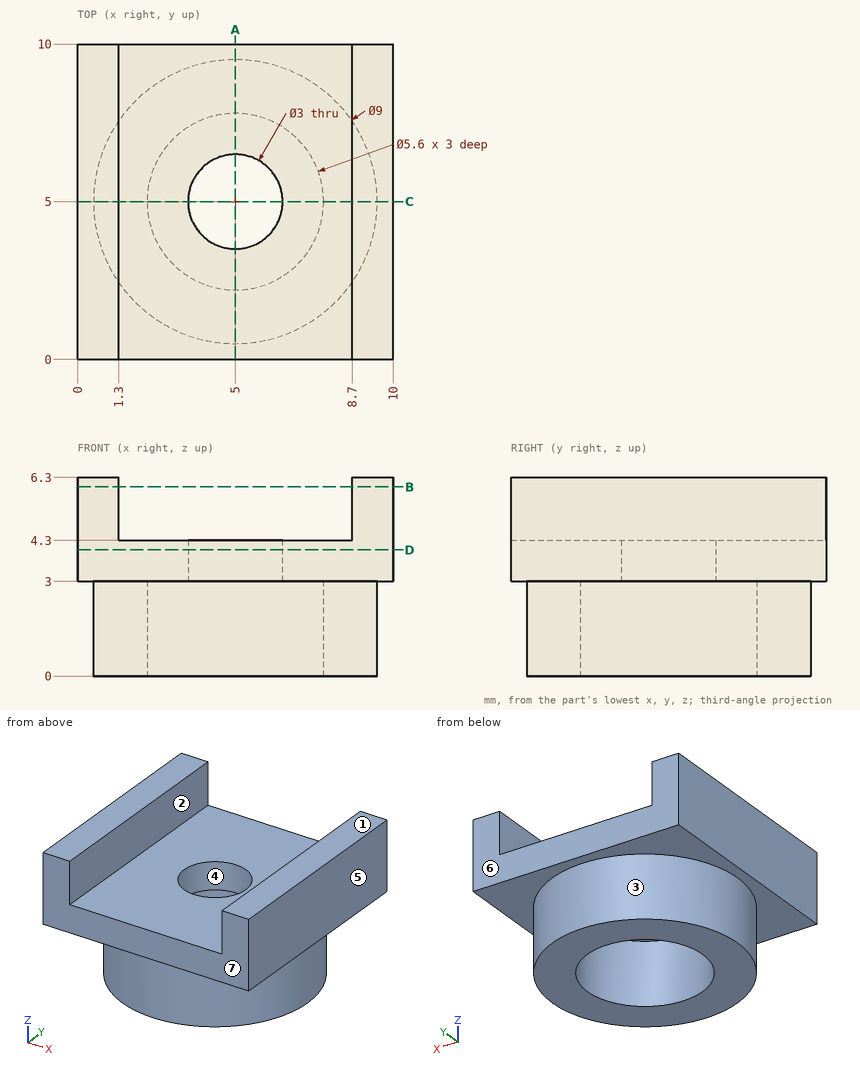
Geometry: see drawing. Coordinates: mm, zero at the bounding-box minimum. A direction names the side the tool comes from. Coordinates: 2 decimals unless noted, no trailing zeros. Loops run counter-clockwise (first coordinate to the right, second up) from the corner with the lowest first, then second, coordinate; pieces in that order, holes last. Notation, with made-up numbers: (36, 6) - (40, 6) arc R23 ccw to (40, 37) - close; hole circle Ø9 at (44, 77.5). An arc over 180 degrees is marked (long way). Answer in a Markdown table with one row per item.
(1) Set-up query: the marked faces 1, 2 and 3. Return all of +Z, -Z, +X, -X, +Y, -Y with unobstructed straight access to the full face (end or side cutting, diameter ignored); none if empty.
Model answer:
| item | result |
|---|---|
| face 1 | +Z, +X, -X, +Y, -Y |
| face 2 | +Z, +Y, -Y |
| face 3 | -Z |
(2) Material intervals for L1, parallel to X at y = 9.5, z = 5.5; L2, parallel to Y at x = 5, z = 2.25; L3, parallel to Y at x = 5, z = 3.6, sorted ascending. Write a range as from..to.
Model answer:
| item | result |
|---|---|
| L1 | x = 0..1.3, 8.7..10 |
| L2 | y = 0.5..2.2, 7.8..9.5 |
| L3 | y = 0..3.5, 6.5..10 |
(3) Cut plane A-A on x = 5. Output: boundary loops of the cut face in (y, z).
Model answer:
| item | result |
|---|---|
| outline | (0, 3) - (0.5, 3) - (0.5, 0) - (2.2, 0) - (2.2, 3) - (3.5, 3) - (3.5, 4.3) - (0, 4.3) - close; (6.5, 3) - (7.8, 3) - (7.8, 0) - (9.5, 0) - (9.5, 3) - (10, 3) - (10, 4.3) - (6.5, 4.3) - close |
(4) Pin query (flat end, axial travel): P1, Ø3.5, axis at x = 6.5, y = 3.5, coming from the +Z side; P2, Ø3, axis at x = 4, y = 6, coming from the -Z side; P3, Ø3.5, axis at x = 5, y = 5, coming from the -Z side; P4, Ø3, axis at x = 8, z = 1, coming from the -Y side. Return the tip coordinate at first contact, or that it passes through.
Model answer:
| item | result |
|---|---|
| P1 | stops at z = 4.3 |
| P2 | stops at z = 0 |
| P3 | stops at z = 3 |
| P4 | stops at y = 0.76 |
(5) Cut plane B-B on z = 6. Output: boundary loops of the cut face in (x, y), plus the area to 3 significant figures.
Model answer:
| item | result |
|---|---|
| outline | (0, 0) - (1.3, 0) - (1.3, 10) - (0, 10) - close; (8.7, 0) - (10, 0) - (10, 10) - (8.7, 10) - close |
| area | 26.0 mm² |
(6) Mould query, pull axis Y, two halves, no side actions, for the marked faces 4, 5, 6 and 7. Classes: pulls with the +Y half, pulls with the -Y half, needs draft (parallel to the pull), parting line crosses it, or undercut.
Model answer:
| item | result |
|---|---|
| face 4 | undercut |
| face 5 | needs draft |
| face 6 | pulls with the +Y half |
| face 7 | pulls with the -Y half |
(7) Cut plane D-D on z = 4. Output: boundary loops of the cut face in (x, y).
Model answer:
| item | result |
|---|---|
| outline | (0, 0) - (10, 0) - (10, 10) - (0, 10) - close; hole circle Ø3 at (5, 5) |
(8) Cut plane C-C on y = 5. Output: boundary loops of the cut face in (x, z).
Model answer:
| item | result |
|---|---|
| outline | (0, 3) - (0.5, 3) - (0.5, 0) - (2.2, 0) - (2.2, 3) - (3.5, 3) - (3.5, 4.3) - (1.3, 4.3) - (1.3, 6.3) - (0, 6.3) - close; (6.5, 3) - (7.8, 3) - (7.8, 0) - (9.5, 0) - (9.5, 3) - (10, 3) - (10, 6.3) - (8.7, 6.3) - (8.7, 4.3) - (6.5, 4.3) - close |
